from build123d import *

# Parameters (mm, degrees)
CYLINDER050_R             = 0.9
CYLINDER050_DEPTH         = 7
CYLINDER051_R             = 0.9
CYLINDER051_DEPTH         = 7
CYLINDER043_R             = 0.95
CYLINDER043_DEPTH         = 10
CYLINDER044_R             = 0.95
CYLINDER044_DEPTH         = 10
CYLINDER041_R             = 0.95
CYLINDER041_DEPTH         = 10
CYLINDER042_R             = 0.95
CYLINDER042_DEPTH         = 10
BOX007_W                  = 10
BOX007_H                  = 10
BOX007_DEPTH              = 7
PAD016_DEPTH              = 21
CYLINDER040_R             = 3
CYLINDER040_DEPTH         = 10
CYLINDER048_R             = 0.95
CYLINDER048_DEPTH         = 10
CYLINDER049_R             = 0.95
CYLINDER049_DEPTH         = 10
CYLINDER046_R             = 0.95
CYLINDER046_DEPTH         = 10
CYLINDER047_R             = 0.95
CYLINDER047_DEPTH         = 10
BOX008_W                  = 10
BOX008_H                  = 10
BOX008_DEPTH              = 7
PAD017_DEPTH              = 21
CYLINDER045_R             = 3
CYLINDER045_DEPTH         = 10
FUSION040_PLACEMENT_ANGLE = 180


with BuildPart() as cylinder050:
    # Cylinder050 → Cylinder050 (new body)
    with BuildSketch(Plane(origin=(7, 28.5, 25), x_dir=(0, 0, 1), z_dir=(-1, 0, 0))):
        Circle(CYLINDER050_R)
    extrude(amount=CYLINDER050_DEPTH)


with BuildPart() as fusion042:
    # Cylinder051 → Cylinder051 (new body)
    with BuildSketch(Plane(origin=(7, 28.5, 5), x_dir=(0, 0, 1), z_dir=(-1, 0, 0))):
        Circle(CYLINDER051_R)
    extrude(amount=CYLINDER051_DEPTH)

    # Fusion042: union Cylinder050
    add(cylinder050.part)


with BuildPart() as cylinder043:
    # Cylinder043 → Cylinder043 (new body)
    with BuildSketch(Plane(origin=(9.9, 0, 0), x_dir=(1, 0, 0), z_dir=(0, 0, 1))):
        Circle(CYLINDER043_R)
    extrude(amount=CYLINDER043_DEPTH)


with BuildPart() as tornillos015:
    # Cylinder044 → Cylinder044 (new body)
    with BuildSketch(Plane.XY):
        Circle(CYLINDER044_R)
    extrude(amount=CYLINDER044_DEPTH)

    # Fusion034: union Cylinder043
    add(cylinder043.part)


with BuildPart() as tornillos015_1:
    # Fusion034 placement: moved
    add(tornillos015.part.moved(Location((5, -24.5, 22))))


with BuildPart() as cylinder041:
    # Cylinder041 → Cylinder041 (new body)
    with BuildSketch(Plane(origin=(9.9, 0, 0), x_dir=(1, 0, 0), z_dir=(0, 0, 1))):
        Circle(CYLINDER041_R)
    extrude(amount=CYLINDER041_DEPTH)


with BuildPart() as fusion035:
    # Cylinder042 → Cylinder042 (new body)
    with BuildSketch(Plane.XY):
        Circle(CYLINDER042_R)
    extrude(amount=CYLINDER042_DEPTH)

    # Fusion033: union Cylinder041
    add(cylinder041.part)


with BuildPart() as fusion035_1:
    # Fusion033 placement: moved
    add(fusion035.part.moved(Location((5, 24.5, 22))))

    # Fusion035: union Tornillos015
    add(tornillos015_1.part)


with BuildPart() as fusion035_2:
    # Fusion035 placement: moved
    add(fusion035_1.part.moved(Location((0.4, 0, 0))))


with BuildPart() as cube007:
    # Box007 → Box007 (new body)
    with BuildSketch(Plane(origin=(5, -29, 7), x_dir=(1, 0, 0), z_dir=(0, 0, 1))):
        with Locations((5, 5)):
            Rectangle(BOX007_W, BOX007_H)
    extrude(amount=BOX007_DEPTH)


with BuildPart() as holder008:
    # Sketch016 → Pad016 (new body)
    with BuildSketch(Plane.YZ):
        Polygon((-28.75, 32), (-28.75, 0), (28.75, 0), (28.75, 32), (20.75, 32), (20.75, 3.5), (-20.75, 3.5), (-20.75, 32), align=None)
    extrude(amount=PAD016_DEPTH)

    # Cut022: cut Cube007
    add(cube007.part, mode=Mode.SUBTRACT)

    # Cut023: cut Fusion035
    add(fusion035_2.part, mode=Mode.SUBTRACT)


with BuildPart() as obj1:
    # Cylinder040 → Cylinder040 (new body)
    with BuildSketch(Plane(origin=(10.5, -10.1, -7), x_dir=(1, 0, 0), z_dir=(0, 0, 1))):
        Circle(CYLINDER040_R)
    extrude(amount=CYLINDER040_DEPTH)

    # Fusion036: union Holder008
    add(holder008.part)


with BuildPart() as cylinder048:
    # Cylinder048 → Cylinder048 (new body)
    with BuildSketch(Plane(origin=(9.9, 0, 0), x_dir=(1, 0, 0), z_dir=(0, 0, 1))):
        Circle(CYLINDER048_R)
    extrude(amount=CYLINDER048_DEPTH)


with BuildPart() as tornillos017:
    # Cylinder049 → Cylinder049 (new body)
    with BuildSketch(Plane.XY):
        Circle(CYLINDER049_R)
    extrude(amount=CYLINDER049_DEPTH)

    # Fusion038: union Cylinder048
    add(cylinder048.part)


with BuildPart() as tornillos017_1:
    # Fusion038 placement: moved
    add(tornillos017.part.moved(Location((5, -24.5, 22))))


with BuildPart() as cylinder046:
    # Cylinder046 → Cylinder046 (new body)
    with BuildSketch(Plane(origin=(9.9, 0, 0), x_dir=(1, 0, 0), z_dir=(0, 0, 1))):
        Circle(CYLINDER046_R)
    extrude(amount=CYLINDER046_DEPTH)


with BuildPart() as fusion039:
    # Cylinder047 → Cylinder047 (new body)
    with BuildSketch(Plane.XY):
        Circle(CYLINDER047_R)
    extrude(amount=CYLINDER047_DEPTH)

    # Fusion037: union Cylinder046
    add(cylinder046.part)


with BuildPart() as fusion039_1:
    # Fusion037 placement: moved
    add(fusion039.part.moved(Location((5, 24.5, 22))))

    # Fusion039: union Tornillos017
    add(tornillos017_1.part)


with BuildPart() as fusion039_2:
    # Fusion039 placement: moved
    add(fusion039_1.part.moved(Location((0.4, 0, 0))))


with BuildPart() as cube008:
    # Box008 → Box008 (new body)
    with BuildSketch(Plane(origin=(5, -29, 7), x_dir=(1, 0, 0), z_dir=(0, 0, 1))):
        with Locations((5, 5)):
            Rectangle(BOX008_W, BOX008_H)
    extrude(amount=BOX008_DEPTH)


with BuildPart() as holder009:
    # Sketch017 → Pad017 (new body)
    with BuildSketch(Plane.YZ):
        Polygon((-28.75, 32), (-28.75, 0), (28.75, 0), (28.75, 32), (20.75, 32), (20.75, 3.5), (-20.75, 3.5), (-20.75, 32), align=None)
    extrude(amount=PAD017_DEPTH)

    # Cut024: cut Cube008
    add(cube008.part, mode=Mode.SUBTRACT)

    # Cut025: cut Fusion039
    add(fusion039_2.part, mode=Mode.SUBTRACT)


with BuildPart() as cut026:
    # Cylinder045 → Cylinder045 (new body)
    with BuildSketch(Plane(origin=(10.5, -10.1, -7), x_dir=(1, 0, 0), z_dir=(0, 0, 1))):
        Circle(CYLINDER045_R)
    extrude(amount=CYLINDER045_DEPTH)

    # Fusion040: union Holder009
    add(holder009.part)


with BuildPart() as cut026_1:
    # Fusion040 placement: moved
    add(cut026.part.moved(Location((21, 57, 0))).rotate(Axis((21, 57, 0), (0, 0, 1)), FUSION040_PLACEMENT_ANGLE))

    # Fusion041: union obj1
    add(obj1.part)

    # Cut026: cut Fusion042
    add(fusion042.part, mode=Mode.SUBTRACT)


solid = cut026_1.part
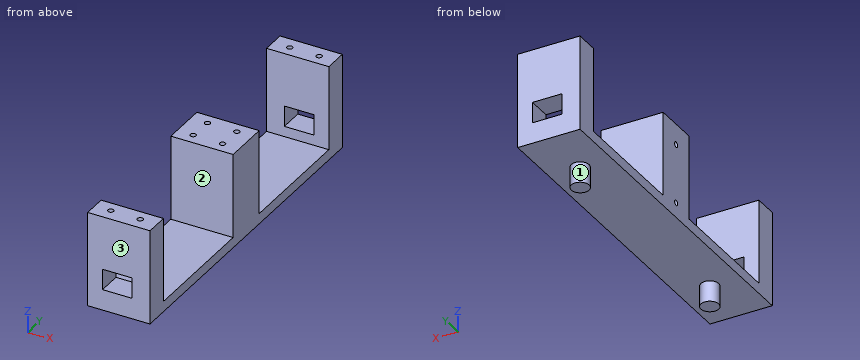
Check sheet for the modelled part. Datum: model origin and axes. Units: mm. Face numbers are marked on the shaded views. A direction names the side the tool comes from. Round coordinates to 2 decimals unless told otherwise and drop trailing zeros. Order: outer loops, then holes, each group sorted by start corner. A loop starts at its lowest first (then second) coordinate and runs counter-clockwise, first axis right, second up. Notation, with made-up numbers: M 30.5,79.25 L 39.5,79.25 A5 ccw 39.5,88.25 Z; hole C 2,-27 d4. An arc over 180 degrees is marked long. One line per item, written item: value. Start each with the question number.
1. Section check A-A on z = 17. Enter the section's corners in (x, y), and give its area (4 significant figures).
2. Access from +Z, -Z, +X, -X, +Y, -Y to the whole of each face (thin tool, end or side, straight path). Record for the marked faces 1, 2 and 3.
3. Section check D-D on x = 3. Enter the section's corners in (y, z).
4. Section check B-B on x = 10. Enter the section's corners in (y, z).
5. Scan lines: line 1 along Y through (x, z) = (2.5, 9.5); line 2 along X through (y, z) = (81, 25); line 3 along Z through (x, y) = (4.75, 71.5). Record each from-to range of solid material in increasing order.
6. Section check C-C on z = 9.5. Enter the section's corners in (x, y).
7. Gauge pin test, flat ends, axial feed: P1, Ø5, axis at x = 14.5, y = 74, coming from the +Z side; P2, Ø1.7, axis at x = 5.4, y = 24.5, coming from the +Z side; P3, Ø2, axis at x = 17, y = 20.5, coming from the -Z side; P4, Ø5, axis at y = 43.5, z = -2, coming from the -X side. Record the tip position at first contact, or that the pin passes through.
Results found:
1. outline: M 0,-28.75 L 21,-28.75 L 21,-20.75 L 0,-20.75 Z; M 0,20.75 L 21,20.75 L 21,36.25 L 0,36.25 Z; M 0,77.75 L 21,77.75 L 21,85.75 L 0,85.75 Z
1. area: 661.5 mm^2
2. face 1: -Z
2. face 2: +Z, +X, -X
2. face 3: +Z, -Z, +X, -X, -Y
3. outline: M -28.75,0 L 85.75,0 L 85.75,32 L 77.75,32 L 77.75,3.5 L 36.25,3.5 L 36.25,32 L 20.75,32 L 20.75,3.5 L -20.75,3.5 L -20.75,32 L -28.75,32 Z; hole C 28.5,5 d1.8; hole C 28.5,25 d1.8
4. outline: M -28.75,0 L -13.06,0 L -13.06,-7 L -7.14,-7 L -7.14,0 L 64.14,0 L 64.14,-7 L 70.06,-7 L 70.06,0 L 85.75,0 L 85.75,7 L 77.75,7 L 77.75,3.5 L 36.25,3.5 L 36.25,32 L 20.75,32 L 20.75,3.5 L -20.75,3.5 L -20.75,7 L -28.75,7 Z; M -28.75,14 L -20.75,14 L -20.75,32 L -28.75,32 Z; M 77.75,14 L 85.75,14 L 85.75,32 L 77.75,32 Z
5. line 1: -28.75 to -20.75, 20.75 to 36.25, 77.75 to 85.75
5. line 2: 0 to 4.89, 6.51 to 14.79, 16.41 to 21
5. line 3: 0 to 3.5
6. outline: M 0,-28.75 L 5,-28.75 L 5,-20.75 L 0,-20.75 Z; M 0,20.75 L 21,20.75 L 21,36.25 L 0,36.25 Z; M 0,77.75 L 6,77.75 L 6,85.75 L 0,85.75 Z; M 15,-28.75 L 21,-28.75 L 21,-20.75 L 15,-20.75 Z; M 16,77.75 L 21,77.75 L 21,85.75 L 16,85.75 Z
7. P1: z = 3.5
7. P2: z = 22
7. P3: z = 0
7. P4: x = 0
